Build history of the part. All positions in model axes, mm. A direction names the side the tool comes from. Give positions to 0.01 mm unless a question says otherwise; leave off trailing zeros. Loops run counter-clockwise (first coordinate to the right, second up) from the corner with the lowest first, then second, coordinate; pieces in that order, holes last. Notation, with made-up numbers: (66, 23) - (79, 23) arc R22 cw to (79, 40) - close; hole circle Ø11 at (85.5, -24). An arc over 180 degrees is marked (long way). Return JSON: item names as keys, results as strings. Group by question number.
1) Mould opens along X. For faces 1 (the face through (1.284, 0.493, -7.247)), 2 (the face through (-1, 1, -1)), 3 (the face through (-99, 0.507, -55.434)), 4 (the face through (0.9, 0.5, -37.2)) say: released by +X, released by -X, zero draft, split by the parting line, or undercut.
2) Slice it at A-A (z = -26). List the corners of the cut face in (x, y), and give its area (3 significant figures).
3) 3-axis set-ups, long thin cutter, end or side, ignore diameter. For faces 5 (the face through (50.416, 0.493, 40.539)), 6 (the face through (-1, 0, -1)): which of +Z, -Z, +X, -X, +Y, -Y reach the whole face in a straight line?
4) Drill centre lines: probe 1 along Z at (x, y) = (-59.5, 0.65) (3 decimals); probe 2 along Z at (x, y) = (59.5, 0.85) (3 decimals); probe 3 along Z at (x, y) = (12.5, 0.85) (1 decimal). Where is each one in solid material? Low to high. Write a range as from..to.
5) Drop a flat-ended pin along its axis: pin 1 (1.6 mm diameter, centred on x = 60.8, z = 32.895, fed in from +Y). Give the stop position or say it passes through.
6) Slice it at B-B (y = 0.4). Count the separate pieces of the cut face and the enclosed holes in it, and give its area (3 significant figures).
```python
from build123d import *

# Parameters (mm, degrees)
SKETCH1_W           = 205.38
SKETCH1_H           = 118.65
SKETCH1_R           = 4.275
SKETCH1_R_2         = 0.89
BOSS_EXTRUDE1_DEPTH = 1
FILLET1_R           = 12.94


with BuildPart() as part:
    # Sketch1 → Boss-Extrude1 (new body)
    with BuildSketch(Plane(origin=(0, 0, 0), x_dir=(1, 0, 0), z_dir=(0, 1, 0))):
        Rectangle(SKETCH1_W, SKETCH1_H)
        with Locations(Location((0, -40.445, 0), (0, 0, 270))):
            Circle(SKETCH1_R, mode=Mode.SUBTRACT)
        with Locations(Location((-14.35, -40.445, 0), (0, 0, 270))):
            Circle(SKETCH1_R, mode=Mode.SUBTRACT)
        with Locations(Location((0, -32.895, 0), (0, 0, 270))):
            Circle(SKETCH1_R_2, mode=Mode.SUBTRACT)
        with Locations(Location((-14.35, -32.895, 0), (0, 0, 270))):
            Circle(SKETCH1_R_2, mode=Mode.SUBTRACT)
        with Locations(Location((0, 11.325, 0), (0, 0, 270))):
            Circle(SKETCH1_R, mode=Mode.SUBTRACT)
        with Locations(Location((-60.8, 11.325, 0), (0, 0, 270))):
            Circle(SKETCH1_R, mode=Mode.SUBTRACT)
        with Locations(Location((-60.8, -32.895, 0), (0, 0, 270))):
            Circle(SKETCH1_R_2, mode=Mode.SUBTRACT)
        with Locations(Location((14.35, -32.895, 0), (0, 0, 90))):
            Circle(SKETCH1_R_2, mode=Mode.SUBTRACT)
        with Locations(Location((14.35, -40.445, 0), (0, 0, 90))):
            Circle(SKETCH1_R, mode=Mode.SUBTRACT)
        with Locations(Location((60.8, -32.895, 0), (0, 0, 90))):
            Circle(SKETCH1_R_2, mode=Mode.SUBTRACT)
        with Locations(Location((60.8, 11.325, 0), (0, 0, 90))):
            Circle(SKETCH1_R, mode=Mode.SUBTRACT)
        with Locations(Location((-60.8, -40.445, 0), (0, 0, 270))):
            Circle(SKETCH1_R, mode=Mode.SUBTRACT)
        with BuildLine():
            Line((54.69, -36.17), (66.91, -36.17))
            ThreePointArc((66.91, -36.17), (71.185, -40.445), (66.91, -44.72))
            Line((66.91, -44.72), (54.69, -44.72))
            ThreePointArc((54.69, -44.72), (50.415, -40.445), (54.69, -36.17))
        make_face(mode=Mode.SUBTRACT)
        with BuildLine():
            ThreePointArc((18.306994565, -6.981994565), (0, 37.215), (-18.306994565, -6.981994565))
            ThreePointArc((-18.306994565, -6.981994565), (-15.627059864, -6.981994565), (-15.627059864, -4.302059864))
            ThreePointArc((-15.627059864, -4.302059864), (0, 33.425), (15.627059864, -4.302059864))
            ThreePointArc((15.627059864, -4.302059864), (15.627059864, -6.981994565), (18.306994565, -6.981994565))
        make_face(mode=Mode.SUBTRACT)
        with BuildLine():
            ThreePointArc((-42.493005435, -6.981994565), (-45.172940136, -6.981994565), (-45.172940136, -4.302059864))
            ThreePointArc((-45.172940136, -4.302059864), (-60.8, 33.425), (-76.427059864, -4.302059864))
            ThreePointArc((-76.427059864, -4.302059864), (-76.427059864, -6.981994565), (-79.106994565, -6.981994565))
            ThreePointArc((-79.106994565, -6.981994565), (-60.8, 37.215), (-42.493005435, -6.981994565))
        make_face(mode=Mode.SUBTRACT)
        with BuildLine():
            ThreePointArc((42.493005435, -6.981994565), (45.172940136, -6.981994565), (45.172940136, -4.302059864))
            ThreePointArc((45.172940136, -4.302059864), (60.8, 33.425), (76.427059864, -4.302059864))
            ThreePointArc((76.427059864, -4.302059864), (76.427059864, -6.981994565), (79.106994565, -6.981994565))
            ThreePointArc((79.106994565, -6.981994565), (60.8, 37.215), (42.493005435, -6.981994565))
        make_face(mode=Mode.SUBTRACT)
    extrude(amount=BOSS_EXTRUDE1_DEPTH)

    # Fillet1
    fillet1_edges = [part.edges().sort_by_distance(p)[0] for p in [
        (102.69, 0.5, 59.325),
        (-102.69, 0.5, 59.325),
        (-102.69, 0.5, -59.325),
        (102.69, 0.5, -59.325),
    ]]
    fillet(fillet1_edges, radius=FILLET1_R)


solid = part.part
```
Results:
{
 "1": {"face 1": "undercut", "face 2": "zero draft", "face 3": "released by -X", "face 4": "undercut"},
 "2": {"outline": "(-102.69, 0) - (-82.13, 0) - (-82.13, 1) - (-102.69, 1) - close; (-77.32, 0) - (-44.28, 0) - (-44.28, 1) - (-77.32, 1) - close; (-39.47, 0) - (-21.33, 0) - (-21.33, 1) - (-39.47, 1) - close; (-16.52, 0) - (16.52, 0) - (16.52, 1) - (-16.52, 1) - close; (21.33, 0) - (39.47, 0) - (39.47, 1) - (21.33, 1) - close; (44.28, 0) - (77.32, 0) - (77.32, 1) - (44.28, 1) - close; (82.13, 0) - (102.69, 0) - (102.69, 1) - (82.13, 1) - close", "area": "177 mm2"},
 "3": {"face 5": "+Y, -Y", "face 6": "+Z, -Z, +X, -X, -Y"},
 "4": {"probe 1": "-59.325..-37.182, -33.387..-15.398, -7.252..36.372, 44.518..59.325", "probe 2": "-59.325..-37.182, -33.387..-15.398, -7.252..36.17, 44.72..59.325", "probe 3": "-59.3..-34, -29.6..36.6, 44.3..59.3"},
 "5": {"pin 1": "through"},
 "6": {"separate pieces": "1", "enclosed holes": "16", "area": "22,300 mm2"}
}
